The model under review builds one solid part; all positions refer to its coordinate system, in mm. A direction names the side the tool comes from. Coordinates: 2 decimals unless noted, no trailing zeros. Write each loop counter-clockwise with the first axis right and the second up, starting at its lowest first coordinate (ties: lowest second). Pieces come first, ordered by that corner, then holes. Notation, with made-up numbers: (-15.5, 13.5) -> (3.5, 13.5) arc R18 cw to (3.5, 27.5) -> close; hole circle Ø10 at (38, 68.5). An arc over 180 degrees is marked (long way). Write each question's results on one line, items separated by ' | '.
```python
from build123d import *

# Parameters (mm, degrees)
SKETCH_1_W          = 20
SKETCH_1_H          = 20
EXTRUDE_1_DEPTH     = 4
SKETCH_2_W          = 12.9
SKETCH_2_H          = 20
EXTRUDE_2_DEPTH     = 3.8
SKETCH_3_R          = 1.6
CUT_EXTRUDE_1_DEPTH = 30.340074983
SKETCH_4_W          = 5.8
SKETCH_4_H          = 20
SKETCH_4_R          = 1.6
EXTRUDE_3_DEPTH     = 1.5
SKETCH_5_R          = 3
CUT_EXTRUDE_3_DEPTH = 2.4
CHAMFER_3_SIZE      = 1.5
CHAMFER_1_SIZE      = 6.6
CHAMFER_2_SIZE      = 1
CHAMFER_4_SIZE      = 0.4
CHAMFER_5_SIZE      = 0.9
SKETCH_7_W          = 21.061561739
SKETCH_7_H          = 3.8
CUT_EXTRUDE_6_DEPTH = 0.5


with BuildPart() as part:
    # 草图1 → 凸台-拉伸1 (new body)
    with BuildSketch(Plane(origin=(0, 0, 0), x_dir=(1, 0, 0), z_dir=(0, 1, 0))):
        with Locations((10, 10)):
            Rectangle(SKETCH_1_W, SKETCH_1_H)
    extrude(amount=EXTRUDE_1_DEPTH)

    # 草图2 → 凸台-拉伸2 (add)
    with BuildSketch(Plane(origin=(0, 4, 0), x_dir=(1, 0, 0), z_dir=(0, 1, 0))):
        with Locations((6.45, 10)):
            Rectangle(SKETCH_2_W, SKETCH_2_H)
    extrude(amount=EXTRUDE_2_DEPTH)

    # 草图3 → 切除-拉伸1 (cut, through all)
    with BuildSketch(Plane(origin=(0, 0, 0), x_dir=(-1, 0, 0), z_dir=(0, -1, 0))):
        with Locations(Location((-10, 5, 0), (0, 0, 90))):
            Circle(SKETCH_3_R)
        with Locations(Location((-10, 15, 0), (0, 0, 90))):
            Circle(SKETCH_3_R)
    extrude(amount=-CUT_EXTRUDE_1_DEPTH, mode=Mode.SUBTRACT)

    # 草图4 → 凸台-拉伸3 (add)
    with BuildSketch(Plane(origin=(0, 7.8, 0), x_dir=(1, 0, 0), z_dir=(0, 1, 0))):
        with Locations((10, 10)):
            Rectangle(SKETCH_4_W, SKETCH_4_H)
        with Locations(Location((10, 15, 0), (0, 0, 90))):
            Circle(SKETCH_4_R, mode=Mode.SUBTRACT)
        with Locations(Location((10, 5, 0), (0, 0, 90))):
            Circle(SKETCH_4_R, mode=Mode.SUBTRACT)
    extrude(amount=EXTRUDE_3_DEPTH)

    # 草图5 → 切除-拉伸3 (cut)
    with BuildSketch(Plane(origin=(0, 0, 0), x_dir=(-1, 0, 0), z_dir=(0, -1, 0))):
        with Locations(Location((-10, 5, 0), (0, 0, 90))):
            Circle(SKETCH_5_R)
        with Locations(Location((-10, 15, 0), (0, 0, 90))):
            Circle(SKETCH_5_R)
    extrude(amount=-CUT_EXTRUDE_3_DEPTH, mode=Mode.SUBTRACT)

    # 倒角3
    # the kernel refuses this chamfer: 1.5 mm, written as the material it takes off along each edge
    with BuildSketch(Plane(origin=(10, 2.4, -15), x_dir=(0, 0, -1), z_dir=(-1, 0, 0))) as chamfer_3_piece_1_section:
        Polygon((1.6 + CHAMFER_3_SIZE, 0), (1.6, -CHAMFER_3_SIZE), (1.6, 0), align=None)
    chamfer_3_piece_1 = revolve(axis=Axis((10, 2.4, -15), (0, -1, 0)), mode=Mode.PRIVATE)
    chamfer_3_piece_1 = chamfer_3_piece_1 & Plane(origin=(10, 2.4, -15), x_dir=(0, 0, -1), z_dir=(0, -1, 0)) * Cylinder(3, 13, mode=Mode.PRIVATE)
    add(chamfer_3_piece_1, mode=Mode.SUBTRACT)
    with BuildSketch(Plane(origin=(10, 2.4, -5), x_dir=(0, 0, -1), z_dir=(-1, 0, 0))) as chamfer_3_piece_2_section:
        Polygon((1.6 + CHAMFER_3_SIZE, 0), (1.6, -CHAMFER_3_SIZE), (1.6, 0), align=None)
    chamfer_3_piece_2 = revolve(axis=Axis((10, 2.4, -5), (0, -1, 0)), mode=Mode.PRIVATE)
    chamfer_3_piece_2 = chamfer_3_piece_2 & Plane(origin=(10, 2.4, -5), x_dir=(0, 0, -1), z_dir=(0, -1, 0)) * Cylinder(3, 13, mode=Mode.PRIVATE)
    add(chamfer_3_piece_2, mode=Mode.SUBTRACT)

    # 倒角1
    chamfer_1_edges = [part.edges().sort_by_distance(p)[0] for p in [
        (0, 0, -10),
    ]]
    chamfer(chamfer_1_edges, length=CHAMFER_1_SIZE)

    # 倒角2
    chamfer_2_edges = [part.edges().sort_by_distance(p)[0] for p in [
        (20, 4, -10),
        (16.45, 4, 0),
        (12.9, 6.65, 0),
        (12.9, 6.65, -20),
        (16.45, 4, -20),
        (20, 0, -10),
    ]]
    chamfer(chamfer_2_edges, length=CHAMFER_2_SIZE)

    # 倒角4
    chamfer_4_edges = [part.edges().sort_by_distance(p)[0] for p in [
        (0, 7.8, -10),
    ]]
    chamfer(chamfer_4_edges, length=CHAMFER_4_SIZE)

    # 倒角5
    chamfer_5_edges = [part.edges().sort_by_distance(p)[0] for p in [
        (7.1, 9.3, -10),
        (12.9, 9.3, -10),
    ]]
    chamfer(chamfer_5_edges, length=CHAMFER_5_SIZE)

    # 草图7 → 切除-拉伸6 (cut)
    with BuildSketch(Plane(origin=(12.9, 0, 0), x_dir=(0, 0, -1), z_dir=(1, 0, 0))):
        with Locations((9.469219131, 5.9)):
            Rectangle(SKETCH_7_W, SKETCH_7_H)
    extrude(amount=-CUT_EXTRUDE_6_DEPTH, mode=Mode.SUBTRACT)


solid = part.part
```
Q1. Add section B-B (z = -15). Write out the cut boundary in (x, y).
Solution:
outline: (0, 6.6) -> (6.6, 0) -> (7, 0) -> (7, 2.5) -> (8.4, 3.9) -> (8.4, 9.3) -> (8, 9.3) -> (7.1, 8.4) -> (7.1, 7.8) -> (0.4, 7.8) -> (0, 7.4) -> close; (11.6, 3.9) -> (13, 2.5) -> (13, 0) -> (19, 0) -> (20, 1) -> (20, 3) -> (19, 4) -> (12.4, 4) -> (12.4, 7.8) -> (12.9, 7.8) -> (12.9, 8.4) -> (12, 9.3) -> (11.6, 9.3) -> close
Q2. Add section C-C (y = 8.75). Write out the cut boundary in (x, z), plus the area to 3 significant figures.
Solution:
outline: (7.45, -20) -> (11.9, -20) -> (12.55, -19.35) -> (12.55, -0.65) -> (11.9, 0) -> (7.45, 0) -> close; hole circle Ø3.2 at (10, -15); hole circle Ø3.2 at (10, -5) | area: 85.5 mm²
Q3. Machinability: for faces 1 (the flat face through (12.2, 6.2, -19.7)), 2 (the flat face through (15.9, 3.5, -0.5)), 3 (the cylindrical face through (10, 1, -2)), which of the approach directions +Z, -Z, +X, -X, +Y, -Y give a long, thin tool a straight path to every point of the face, cutting with its end or side? Answer none if there is none.
Solution:
face 1: -Z, +X, +Y | face 2: +Z, +X, +Y | face 3: -Y
Q4. Draft analysis for pull direction Z (two halves, no side actions). For faces 4 (the flat face through (12.2, 6.1, -0.3)), 5 (the cylindrical face through (10, 1, -12)), 6 (the flat face through (10, 4, -20)), 7 (the cylindrical face through (10.97, 6.56, -13.73)), state which applies: pulls with the +Z half, pulls with the -Z half, needs draft (parallel to the pull), parting line crosses it, or undercut.
Solution:
face 4: pulls with the +Z half | face 5: undercut | face 6: pulls with the -Z half | face 7: undercut
Q5. Clearance check with flat-ended pins moving along their axes: P1, Ø3, axis at x = 10, z = -15, coming from the -Y side; P2, Ø1.9, axis at y = 6, z = -13, coming from the +X side; P3, Ø0.5, axis at y = 8, z = -15, coming from the -X side; P4, Ø2, axis at x = 2, z = -6, coming from the +Y side. State where each tip first meets the part, or that it passes through.
Solution:
P1: through | P2: x = 12.4 | P3: x = 0.35 | P4: y = 7.8
Q6. Add section D-D (z = -18.75). Write out the cut boundary in (x, y), plus the area to 3 significant figures.
Solution:
outline: (0, 6.6) -> (6.6, 0) -> (19, 0) -> (20, 1) -> (20, 3) -> (19, 4) -> (12.4, 4) -> (12.4, 7.8) -> (12.9, 7.8) -> (12.9, 8.4) -> (12, 9.3) -> (8, 9.3) -> (7.1, 8.4) -> (7.1, 7.8) -> (0.4, 7.8) -> (0, 7.4) -> close | area: 112 mm²
Q7. For line 1 (Z direction, x = 10, y = 5.9); line 2 (Z direction, x = 8.5, y = 3.75); line 3 (X direction, y = 6.75, z = -5), list the stretches that pass through material, from the lowest coordinate up. Write a range as from..to.
Solution:
line 1: -20..-16.6, -13.4..-6.6, -3.4..0 | line 2: -20..-15.9, -14.1..-5.9, -4.1..0 | line 3: 0..8.4, 11.6..12.4
Q8. Add section A-A (x = 10). Write out the cut boundary in (y, z), plus the area to 3 significant figures.
Solution:
outline: (0, -20) -> (9.3, -20) -> (9.3, -16.6) -> (3.9, -16.6) -> (2.5, -18) -> (0, -18) -> close; (0, -12) -> (2.5, -12) -> (3.9, -13.4) -> (9.3, -13.4) -> (9.3, -6.6) -> (3.9, -6.6) -> (2.5, -8) -> (0, -8) -> close; (0, -2) -> (2.5, -2) -> (3.9, -3.4) -> (9.3, -3.4) -> (9.3, 0) -> (0, 0) -> close | area: 109 mm²
